Design review of the part built by this model. Coordinates are the model's own, in mm. Face numbers are marked on the shaded views. A direction names the side the tool comes from. Coordinates: 2 decimals unless noted, no trailing zeros. Write each loop counter-clockwise with the first axis right and the second up, starting at its lowest first coordinate (ties: lowest second). Pieces come first, ordered by that corner, then holes.
Q1. For L1, parallel to Z at x = 133.5, y = 5.9; L2, parallel to X at y = 5.8, z = -6.5; L3, parallel to Z at x = 43, y = 19.25, list the stretches that pass through material, from the lowest coordinate up.
Q2. Take a section at B-B, the plane x = 133.5. Write out the cut boundary in (y, z).
Q3. Take a section at D-D, the plane x = 87. Write out the cut boundary in (y, z).
Q4. The part is to be moulded in two halves that separate along X. For the marked faces 1, 2 and 3, say which applies: released by +X, released by -X, zero draft, split by the parting line, or undercut.
Q5. Take a section at C-C, the plane z = -35. Write out the cut boundary in (x, y), plus the area to 3 significant figures.
Q6. For pin 1 Ø1.5 at (x, y) = (109.5, 18.5) entering from -Z; pin 2 Ø12.5 at (x, z) = (85, -37) entering from +Y; pin 3 Ø6 at (x, y) = (87, 14) entering from +Z, all flat-tipped, find the tip position at first contact; note any pin that passes through.
Q7. Take a section at A-A, the plane z = -61.5. Write out the cut boundary in (x, y), plus the area to 3 significant figures.
Q8. For the marked faces 4, 5 and 6, list the 3-axis set-ups (+Z, -Z, +X, -X, +Y, -Y) from which the entire face can be reached by the end or side of a thin tool; tool diameter is ignored.
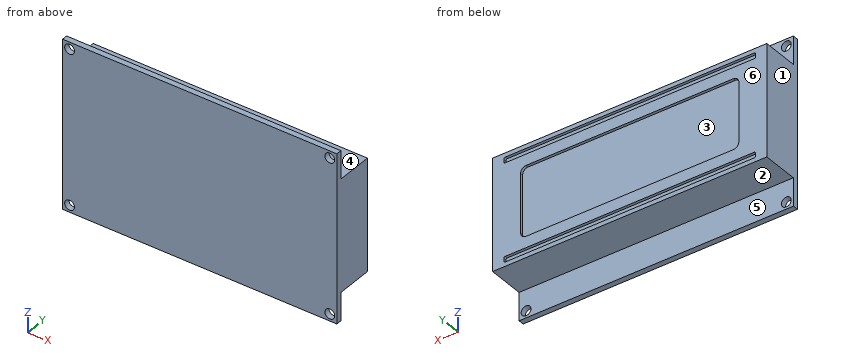
from build123d import *

# Parameters (mm, degrees)
SKETCH1_W               = 150
SKETCH1_H               = 55
SKETCH1_R               = 1.5
BOSS_EXTRUDE1_DEPTH     = 2
SKETCH2_R               = 6
BOSS_EXTRUDE2_DEPTH     = 10
SKETCH3_W               = 12
SKETCH3_H               = 12
BOSS_EXTRUDE3_DEPTH     = 25
SKETCH4_W               = 5
SKETCH4_H               = 5
SKETCH4_W_2             = 41
SKETCH4_H_2             = 3
BOSS_EXTRUDE4_DEPTH     = 5
SKETCH5_W               = 41
SKETCH5_H               = 3
SKETCH5_W_2             = 5
SKETCH5_H_2             = 5
SKETCH5_R               = 1.5
CUT_EXTRUDE1_DEPTH      = 2
SKETCH6_W               = 12
SKETCH6_H               = 12
CUT_EXTRUDE2_DEPTH      = 13
SKETCH7_W               = 12
SKETCH7_H               = 12
SKETCH7_R               = 3.5
CUT_EXTRUDE3_DEPTH      = 7
SKETCH8_R               = 1.25
CUT_EXTRUDE4_DEPTH      = 5
BOSS_EXTRUDE5_DEPTH     = 3
SKETCH10_W              = 25
SKETCH10_H              = 1.5
CUT_EXTRUDE5_DEPTH      = 18
SKETCH11_W              = 98
SKETCH11_H              = 60
SKETCH11_R              = 1.75
BOSS_EXTRUDE6_DEPTH     = 2
SKETCH12_W              = 98
SKETCH12_H              = 40
BOSS_EXTRUDE7_DEPTH     = 13
CUT_EXTRUDE6_DEPTH      = 1
SKETCH14_W              = 25
SKETCH14_H              = 1.5
BOSS_EXTRUDE8_DEPTH     = 29
CUT_EXTRUDE7_DEPTH      = 76
CUT_EXTRUDE7_DEPTH_BACK = 10
SKETCH16_W              = 98
SKETCH16_H              = 8
CUT_EXTRUDE8_DEPTH      = 69


with BuildPart() as part:
    # Sketch1 → Boss-Extrude1 (new body)
    with BuildSketch(Plane(origin=(0, 0, 0), x_dir=(1, 0, 0), z_dir=(0, 1, 0))):
        with Locations((75, 27.5)):
            Rectangle(SKETCH1_W, SKETCH1_H)
        with Locations((3, 52)):
            Circle(SKETCH1_R, mode=Mode.SUBTRACT)
        with Locations((147, 52)):
            Circle(SKETCH1_R, mode=Mode.SUBTRACT)
        with Locations((147, 3)):
            Circle(SKETCH1_R, mode=Mode.SUBTRACT)
        with Locations((3, 3)):
            Circle(SKETCH1_R, mode=Mode.SUBTRACT)
    extrude(amount=BOSS_EXTRUDE1_DEPTH)

    # Sketch2 → Boss-Extrude2 (add)
    with BuildSketch(Plane(origin=(0, 2, 0), x_dir=(1, 0, 0), z_dir=(0, 1, 0))):
        with Locations((13, 10)):
            Circle(SKETCH2_R)
    extrude(amount=BOSS_EXTRUDE2_DEPTH)

    # Sketch3 → Boss-Extrude3 (add)
    with BuildSketch(Plane(origin=(0, 2, 0), x_dir=(1, 0, 0), z_dir=(0, 1, 0))):
        with Locations((13, 27.5)):
            Rectangle(SKETCH3_W, SKETCH3_H)
    extrude(amount=BOSS_EXTRUDE3_DEPTH)

    # Sketch4 → Boss-Extrude4 (add)
    with BuildSketch(Plane(origin=(0, 2, 0), x_dir=(1, 0, 0), z_dir=(0, 1, 0))):
        with Locations((13, 43)):
            Rectangle(SKETCH4_W, SKETCH4_H)
        with Locations((106.5, 6.5)):
            Rectangle(SKETCH4_W_2, SKETCH4_H_2)
    extrude(amount=BOSS_EXTRUDE4_DEPTH)

    # Sketch5 → Cut-Extrude1 (cut)
    with BuildSketch(Plane(origin=(0, 7, 0), x_dir=(1, 0, 0), z_dir=(0, 1, 0))):
        with Locations((106.5, 6.5)):
            Rectangle(SKETCH5_W, SKETCH5_H)
        with Locations((13, 43)):
            Rectangle(SKETCH5_W_2, SKETCH5_H_2)
        with Locations((13, 43)):
            Circle(SKETCH5_R, mode=Mode.SUBTRACT)
    extrude(amount=-CUT_EXTRUDE1_DEPTH, mode=Mode.SUBTRACT)

    # Sketch6 → Cut-Extrude2 (cut)
    with BuildSketch(Plane(origin=(0, 27, 0), x_dir=(1, 0, 0), z_dir=(0, 1, 0))):
        with Locations((13, 27.5)):
            Rectangle(SKETCH6_W, SKETCH6_H)
        with BuildLine():
            Line((10.370614338, 26.055586264), (15.629385662, 26.055586264))
            ThreePointArc((15.629385662, 26.055586264), (13, 30.5), (10.370614338, 26.055586264))
        make_face(mode=Mode.SUBTRACT)
    extrude(amount=-CUT_EXTRUDE2_DEPTH, mode=Mode.SUBTRACT)

    # Sketch7 → Cut-Extrude3 (cut)
    with BuildSketch(Plane(origin=(0, 14, 0), x_dir=(1, 0, 0), z_dir=(0, 1, 0))):
        with Locations((13, 27.5)):
            Rectangle(SKETCH7_W, SKETCH7_H)
        with Locations((13, 27.5)):
            Circle(SKETCH7_R, mode=Mode.SUBTRACT)
    extrude(amount=-CUT_EXTRUDE3_DEPTH, mode=Mode.SUBTRACT)

    # Sketch8 → Cut-Extrude4 (cut)
    with BuildSketch(Plane(origin=(0, 12, 0), x_dir=(1, 0, 0), z_dir=(0, 1, 0))):
        with Locations((13, 10)):
            Circle(SKETCH8_R)
    extrude(amount=-CUT_EXTRUDE4_DEPTH, mode=Mode.SUBTRACT)

    # Sketch9 → Boss-Extrude5 (add)
    with BuildSketch(Plane.XZ):
        Polygon((149, -20), (131, -20), (129, -22), (124, -22), (124, -47), (149, -47), align=None)
    extrude(amount=BOSS_EXTRUDE5_DEPTH)

    # Sketch10 → Cut-Extrude5 (cut)
    with BuildSketch(Plane(origin=(149, 0, 0), x_dir=(0, 0, -1), z_dir=(1, 0, 0))):
        with Locations((33.5, -1.5)):
            Rectangle(SKETCH10_W, SKETCH10_H)
    extrude(amount=-CUT_EXTRUDE5_DEPTH, mode=Mode.SUBTRACT)

    # Sketch11 → Boss-Extrude6 (add)
    with BuildSketch(Plane(origin=(0, 5, 0), x_dir=(1, 0, 0), z_dir=(0, 1, 0))):
        with Locations((87, 34)):
            Rectangle(SKETCH11_W, SKETCH11_H)
        with Locations((40.5, 61.5)):
            Circle(SKETCH11_R, mode=Mode.SUBTRACT)
        with Locations((133.5, 61.5)):
            Circle(SKETCH11_R, mode=Mode.SUBTRACT)
        with Locations((133.5, 6.5)):
            Circle(SKETCH11_R, mode=Mode.SUBTRACT)
        with Locations((40.5, 6.5)):
            Circle(SKETCH11_R, mode=Mode.SUBTRACT)
    extrude(amount=BOSS_EXTRUDE6_DEPTH)

    # Sketch12 → Boss-Extrude7 (add)
    with BuildSketch(Plane(origin=(0, 7, 0), x_dir=(1, 0, 0), z_dir=(0, 1, 0))):
        with Locations((87, 34)):
            Rectangle(SKETCH12_W, SKETCH12_H)
    extrude(amount=BOSS_EXTRUDE7_DEPTH)

    # Sketch13 → Cut-Extrude6 (cut)
    with BuildSketch(Plane(origin=(0, 20, 0), x_dir=(1, 0, 0), z_dir=(0, 1, 0))):
        with BuildLine():
            Line((50, 46.5), (124, 46.5))
            ThreePointArc((124, 46.5), (125.414213562, 45.914213562), (126, 44.5))
            Line((126, 44.5), (126, 23.5))
            ThreePointArc((126, 23.5), (125.414213562, 22.085786438), (124, 21.5))
            Line((124, 21.5), (50, 21.5))
            ThreePointArc((50, 21.5), (48.585786438, 22.085786438), (48, 23.5))
            Line((48, 23.5), (48, 44.5))
            ThreePointArc((48, 44.5), (48.585786438, 45.914213562), (50, 46.5))
        make_face()
        with BuildLine():
            Line((42.5, 52.5), (131.5, 52.5))
            ThreePointArc((131.5, 52.5), (131.853553391, 52.353553391), (132, 52))
            Line((132, 52), (132, 51))
            ThreePointArc((132, 51), (131.853553391, 50.646446609), (131.5, 50.5))
            Line((131.5, 50.5), (42.5, 50.5))
            ThreePointArc((42.5, 50.5), (42.146446609, 50.646446609), (42, 51))
            Line((42, 51), (42, 52))
            ThreePointArc((42, 52), (42.146446609, 52.353553391), (42.5, 52.5))
        make_face()
        with BuildLine():
            Line((132, 16), (132, 17))
            ThreePointArc((132, 17), (131.853553391, 17.353553391), (131.5, 17.5))
            Line((131.5, 17.5), (42.5, 17.5))
            ThreePointArc((42.5, 17.5), (42.146446609, 17.353553391), (42, 17))
            Line((42, 17), (42, 16))
            ThreePointArc((42, 16), (42.146446609, 15.646446609), (42.5, 15.5))
            Line((42.5, 15.5), (131.5, 15.5))
            ThreePointArc((131.5, 15.5), (131.853553391, 15.646446609), (132, 16))
        make_face()
    extrude(amount=-CUT_EXTRUDE6_DEPTH, mode=Mode.SUBTRACT)

    # Sketch14 → Boss-Extrude8 (add)
    with BuildSketch(Plane(origin=(131, 0, 0), x_dir=(0, 0, -1), z_dir=(1, 0, 0))):
        with Locations((33.5, -1.5)):
            Rectangle(SKETCH14_W, SKETCH14_H)
    extrude(amount=BOSS_EXTRUDE8_DEPTH)

    # Sketch15 → Cut-Extrude7 (cut, two sides)
    with BuildSketch(Plane(origin=(0, 2, 0), x_dir=(1, 0, 0), z_dir=(0, 1, 0))) as cut_extrude7_sk:
        Polygon((38, 64), (-8.690723281, 64), (-8.690723281, -2.980686498), (38, -2.980686498), (158.556379493, -2.980686498), (158.556379493, 4), (165.16100148, 4), (165.16100148, 64), (136, 64), (136, 4), (38, 4), align=None)
    extrude(amount=CUT_EXTRUDE7_DEPTH, mode=Mode.SUBTRACT)
    extrude(cut_extrude7_sk.sketch, amount=-CUT_EXTRUDE7_DEPTH_BACK, mode=Mode.SUBTRACT)

    # Sketch16 → Cut-Extrude8 (cut)
    with BuildSketch(Plane.XY.offset(-4)):
        with Locations((87, 1)):
            Rectangle(SKETCH16_W, SKETCH16_H)
    extrude(amount=-CUT_EXTRUDE8_DEPTH, mode=Mode.SUBTRACT)


solid = part.part
Responses:
1. L1: z = -64 to -63.25, -59.75 to -8.25, -4.75 to -4
1. L2: x = 38 to 38.75, 42.25 to 131.75, 135.25 to 136
1. L3: z = -54 to -52.5, -50.5 to -17.5, -15.5 to -14
2. outline: (5, -64) - (7, -64) - (7, -63.25) - (5, -63.25) - close; (5, -59.75) - (7, -59.75) - (7, -54) - (20, -54) - (20, -14) - (7, -14) - (7, -8.25) - (5, -8.25) - close; (5, -4.75) - (7, -4.75) - (7, -4) - (5, -4) - close
3. outline: (5, -64) - (7, -64) - (7, -54) - (20, -54) - (20, -52.5) - (19, -52.5) - (19, -50.5) - (20, -50.5) - (20, -46.5) - (19, -46.5) - (19, -21.5) - (20, -21.5) - (20, -17.5) - (19, -17.5) - (19, -15.5) - (20, -15.5) - (20, -14) - (7, -14) - (7, -4) - (5, -4) - close
4. face 1: released by -X
4. face 2: zero draft
4. face 3: undercut
5. outline: (38, 5) - (136, 5) - (136, 20) - (126, 20) - (126, 19) - (48, 19) - (48, 20) - (38, 20) - close
5. area: 1,390 mm2
6. pin 1: stops at z = -54
6. pin 2: stops at y = 19
6. pin 3: stops at z = -14
7. outline: (38, 5) - (38.75, 5) - (38.75, 7) - (38, 7) - close; (42.25, 5) - (131.75, 5) - (131.75, 7) - (42.25, 7) - close; (135.25, 5) - (136, 5) - (136, 7) - (135.25, 7) - close
7. area: 182 mm2
8. face 4: +Z, +X, -X, +Y
8. face 5: -Z, +X, -X, +Y
8. face 6: +Z, -Z, +X, -X, +Y
